Geometry: final body of the model. Coordinates: model frame, mm. A direction names the side the tool comes from. Coordinates: 2 decimals unless noted, no trailing zeros. Order: outer loops, then holes, each group sorted by start corner. A loop starts at its lowest first (then second) coordinate and runs counter-clockwise, first axis right, second up. Notation, with made-up numbers: M -38.5,60.25 L -16.5,60.25 A25 cw -16.5,77.25 Z; hole C 19,-14 d8. An arc over 180 degrees is marked long. Use CSV: the item, a comma, the result in double quotes. Start each with the question number.
Q1. Section query B-B, the plane y = 0. Output: boundary loops of the cut face in (x, z).
Q2. Mould query, pull axis X, two halves, no side actions, for faces 4 (the face through (3.566, -9.22, -28.202)), 5 (the face through (16.6, 24.8, 28.9)), 6 (the face through (10, -6, -30.15)). Classes: +X half, -X half, draft (parallel to the pull), parting line (faces both ways), or undercut.
Q3. First-contact query: P1, Ø1.5, axis at x = 16, z = -10, coming from the -Y side; P2, Ø6, axis at x = 4, z = -26.25, coming from the -Y side; P3, Ø2.5, axis at x = 12.5, z = 1, coming from the -Y side; P4, Ø9, axis at y = 0, z = 0, coming from the +X side. Flat tips, straight axial feed; report the tip coordinate or a pass-through.
Q4. Section query C-C, the plane x = 4. Output: boundary loops of the cut face in (y, z), and give its area (3 significant figures).
Q5. Ray query, probe 1 along Z at (x, y) = (4, -16.5); probe 2 along X at (y, z) = (-18, -26); probe 3 along Y at (x, z) = (5.25, 0). Return the intervals inside material, ascending.
Q6. Section query A-A, the plane z = 0. Output: boundary loops of the cut face in (x, y), and give its area (3 significant figures).
Q7. Section query D-D, the plane z = -16. Output: boundary loops of the cut face in (x, y).
Q8. Access query for faces 1 (the face through (4, -4.15, 26)), 2 (the face through (13, -46, 7.5)), 3 (the face through (8.79, -55.8, -9.79)). Directions: +Z, -Z, +X, -X, +Y, -Y. A direction counts if a zero-diameter tool reaches every point of the face in a straight line with its end or side. Return the directions, or none.
Autodesk Fusion 360 part; units mm, degrees
sketch "Sketch1" plane through (0, 0, 0) normal (1, 0, 0) x (0, 0, -1)
  circle A0 centre (0, 0) radius 5
  line L0 (-30.15, -21.15) -> (30.15, -21.15)
  line L1 (30.15, -21.15) -> (30.15, 21.15)
  line L2 (-30.15, -21.15) -> (-30.15, 26.15)
  line L3 (-30.15, 26.15) -> (30.15, 26.15)
  line L4 (30.15, 26.15) -> (30.15, 21.15)
  dimension "d11" = 10
  dimension "d127" = 60.3
  dimension "d142" = 21.15
  dimension "d143" = 30.15
extrude "Extrude1" add sketch "Sketch1" along normal blind 8
sketch "Sketch16" plane through (0, -21.15, 0) normal (0, -1, 0) x (1, 0, 0)
  line L0 (0, 30.15) -> (0, -30.15)
  line L1 (0, -30.15) -> (8, -30.15)
  line L2 (8, -30.15) -> (8, 30.15)
  line L3 (8, 30.15) -> (0, 30.15)
  line L4 (4, 26.25) -> (4, -26.25) construction
  circle A0 centre (4, 26.25) radius 2.6
  circle A1 centre (4, -26.25) radius 2.6
  dimension "d144" = 4
  dimension "d145" = 52.5
  dimension "d146" = 5.2
  dimension "d147" = 5.2
  dimension "d148" = 26.25
extrude "Extrude17" cut sketch "Sketch16" against normal blind 7 contours A0 | A1
sketch "Sketch17" plane through (0, -14.15, 0) normal (0, -1, 0) x (1, 0, 0)
  circle A0 centre (4, 26.25) radius 2.6
  line L0 (4, 26.25) -> (4, -26.25)
  circle A1 centre (4, 26.25) radius 2
  circle A2 centre (4, -26.25) radius 2
  dimension "d151" = 52.5
  dimension "d152" = 4
  dimension "d153" = 4
extrude "Extrude18" cut sketch "Sketch17" against normal blind 10 contours A1 | A2
extrude "Extrude19" add 1 faces at (8, 1.9151, -21.7481) along direction (1, 0, 0) blind 10
sketch "Sketch18" plane through (0, -21.15, 0) normal (0, -1, 0) x (1, 0, 0)
  circle A0 centre (4, 26.25) radius 2.6
  circle A1 centre (4, -26.25) radius 2.6
  line L0 (0, 30.15) -> (0, -30.15)
  line L1 (0, -30.15) -> (18, -30.15)
  line L2 (18, -30.15) -> (18, 30.15)
  line L3 (18, 30.15) -> (0, 30.15)
  line L4 (18, 30.15) -> (8, 30.15)
  line L5 (8, 30.15) -> (8, -30.15)
  line L6 (8, -30.15) -> (18, -30.15)
  line L7 (18, -30.15) -> (18, 30.15)
  dimension "d159" = 10
extrude "Extrude20" add sketch "Sketch18" along normal blind 37 contours L1 L2 L3 L4 L5 L6 L7
sketch "Sketch19" plane through (18, 0, 0) normal (1, 0, 0) x (0, 0, -1)
  circle A0 centre (0, 0) radius 5
  line L0 (30.15, -58.15) -> (30.15, 26.15)
  line L1 (30.15, 26.15) -> (-30.15, 26.15)
  line L2 (-30.15, 26.15) -> (-30.15, -58.15)
  line L3 (-7.5, -58.15) -> (7.5, -58.15)
  line L4 (7.5, -53.15) -> (7.5, -38.15)
  line L5 (2.5, -33.15) -> (-2.5, -33.15)
  line L6 (-7.5, -38.15) -> (-7.5, -53.15)
  line L7 (12.5, -58.15) -> (26.15, -58.15)
  line L8 (30.15, -54.15) -> (30.15, 26.15)
  line L9 (30.15, 26.15) -> (-30.15, 26.15)
  line L10 (-30.15, 26.15) -> (-30.15, -54.15)
  arc A1 (-2.5, -33.15) -> (-7.5, -38.15) centre (-2.5, -38.15) ccw
  arc A2 (7.5, -38.15) -> (2.5, -33.15) centre (2.5, -38.15) ccw
  arc A3 (7.5, -53.15) -> (12.5, -58.15) centre (12.5, -53.15) ccw
  line L11 (-26.15, -58.15) -> (-12.5, -58.15)
  arc A4 (-12.5, -58.15) -> (-7.5, -53.15) centre (-12.5, -53.15) ccw
  line L12 (30.15, -58.15) -> (-30.15, -58.15)
  arc A5 (-30.15, -54.15) -> (-26.15, -58.15) centre (-26.15, -54.15) ccw
  arc A6 (26.15, -58.15) -> (30.15, -54.15) centre (26.15, -54.15) ccw
  dimension "d162" = 15
  dimension "d163" = 25
  dimension "d164" = 7.5
  dimension "d165" = 5
  dimension "d166" = 5
  dimension "d167" = 4
  dimension "d168" = 4
extrude "Extrude21" cut sketch "Sketch19" against normal up to surface (10 mm away) contours L0 L12 A6 | L3 L4 L5 L6 A1 A2 A3 A4 L12 | L2 L12 A5
chamfer "Chamfer1" distance 2 angle 45 32 edges at (18, 26.15, 0) (9, 26.15, 30.15) (0, 26.15, 0) (0, 2.5, 30.15) (18, -14, 30.15) (18, -56.9784, 28.9784) (18, -58.15, 19.325) (18, -56.6855, 8.9645) (18, -45.65, 7.5) (18, -34.6145, 6.0355) (18, -33.15, 0) (18, -34.6145, -6.0355) (18, -45.65, -7.5) (18, -56.6855, -8.9645) (18, -58.15, -19.325) (18, -56.9784, -28.9784) (18, -14, -30.15) (8, -37.65, 30.15) (8, -56.9784, 28.9784) (8, -58.15, 19.325) (8, -56.6855, 8.9645) (8, -45.65, 7.5) (8, -34.6145, 6.0355) (8, -33.15, 0) (8, -34.6145, -6.0355) (8, -45.65, -7.5) (8, -56.6855, -8.9645) (8, -58.15, -19.325) (8, -56.9784, -28.9784) (8, -37.65, -30.15) (0, 2.5, -30.15) (9, 26.15, -30.15)
equation "d143 = ( 60.3 / 2 ) * 1 mm"
equation "d148 = ( 52.5 / 2 ) * 1 mm"
Responses:
1,outline,"M 0,-28.15 L 2,-30.15 L 16,-30.15 L 18,-28.15 L 18,-5 L 0,-5 Z; M 0,5 L 18,5 L 18,28.15 L 16,30.15 L 2,30.15 L 0,28.15 Z"
2,face 4,"undercut"
2,face 5,"+X half"
2,face 6,"draft"
3,P1,"stops at y = -57.83"
3,P2,"stops at y = -21.15"
3,P3,"stops at y = -33.15"
3,P4,"passes through"
4,outline,"M -21.15,-30.15 L 24.15,-30.15 L 26.15,-28.15 L 26.15,28.15 L 24.15,30.15 L -21.15,30.15 L -21.15,28.85 L -14.15,28.85 L -14.15,28.25 L -4.15,28.25 L -4.15,24.25 L -14.15,24.25 L -14.15,23.65 L -21.15,23.65 L -21.15,-23.65 L -14.15,-23.65 L -14.15,-24.25 L -4.15,-24.25 L -4.15,-28.25 L -14.15,-28.25 L -14.15,-28.85 L -21.15,-28.85 Z; hole C 0,0 d10"
4,area,"2,620 mm²"
5,probe 1,"z = -30.15 to -28.85, -23.65 to 23.65, 28.85 to 30.15"
5,probe 2,"x = 0 to 1.41, 6.59 to 18"
5,probe 3,"y = -21.15 to -5, 5 to 26.15"
6,outline,"M 0,-21.15 L 8,-21.15 L 8,-31.15 L 10,-33.15 L 16,-33.15 L 18,-31.15 L 18,-5 L 0,-5 Z; M 0,5 L 18,5 L 18,24.15 L 16,26.15 L 2,26.15 L 0,24.15 Z"
6,area,"783 mm²"
7,outline,"M 0,-21.15 L 8,-21.15 L 8,-56.15 L 10,-58.15 L 16,-58.15 L 18,-56.15 L 18,24.15 L 16,26.15 L 2,26.15 L 0,24.15 Z"
8,face 1,"-Y"
8,face 2,"+X, -X, -Y"
8,face 3,"-X, -Y"
